from build123d import *

# Parameters (mm, degrees)
PAD_DEPTH    = 0.245
SKETCH003_R  = 0.495763
PAD001_DEPTH = 12.96675


with BuildPart() as part:
    # Sketch → Pad (new body, symmetric)
    with BuildSketch(Plane.XY):
        with BuildLine():
            Line((0, 0.375), (14.4075, 0.375))
            ThreePointArc((14.4075, -0.375), (14.7825, 0), (14.4075, 0.375))
            Line((14.4075, -0.375), (0, -0.375))
            Line((0, 0), (0, -0.375))
            Line((0, 0.375), (0, 0))
        make_face()
    extrude(amount=PAD_DEPTH, both=True)

    # Sketch002 → Revolution001 (revolve)
    with BuildSketch(Plane.XY):
        with BuildLine():
            ThreePointArc((14.4075, -0.625), (15.0325, 0), (14.4075, 0.625))
            Line((14.4075, 0.625), (14.4075, 0))
            Line((14.4075, 0), (14.4075, -0.625))
        make_face()
    revolve(axis=Axis((14.4075, 0, 0), (0, -1, 0)))

    # Sketch003 → Pad001 (join)
    with BuildSketch(Plane.YZ):
        Circle(SKETCH003_R)
    extrude(amount=PAD001_DEPTH)


solid = part.part
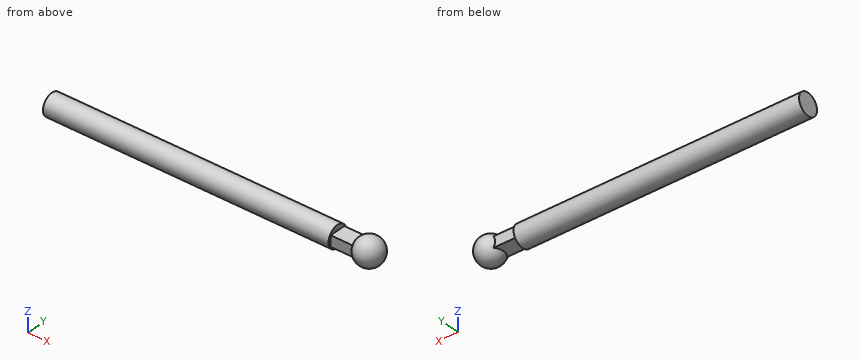
Model file for the job. Use its own axes, mm. Round coordinates to 2 decimals unless told otherwise and drop trailing zeros. Loops run counter-clockwise (first coordinate to the right, second up) from the corner with the lowest first, then second, coordinate; pieces in that order, holes last. Notation, with made-up numbers: (76.5, -24) -> (89.5, -24) arc R20 ccw to (89.5, -5) -> close; hole circle Ø3 at (-30, 66.5). An arc over 180 degrees is marked (long way). Answer as CSV lines item,"result". Start each with the question number.
1) Pin check, flat tip, straight feed: P1, Ø0.5, axis at x = 13.5, z = 0, coming from the -Y side (3 decimals). Stop position of the tip, or through.
2) Probe line 1 along Z through (x, y) = (4, -0.05); line 2 along X through (y, z) = (0, -0.4). List the from-to ranges inside material, lowest first.
3) Slice it at A-A (x = 7.75). List the corners of the cut face in (y, z), plus the area to 3 significant figures.
Filled in:
1,P1,"stops at y = -0.375"
2,line 1,"z = -0.49 to 0.49"
2,line 2,"x = 0 to 12.97, 13.93 to 14.89"
3,outline,"circle Ø0.99 at (0, 0)"
3,area,"0.772 mm2"
